```python
from build123d import *

# Parameters (mm, degrees)
SKETCH1_R           = 4
SKETCH1_R_2         = 1.5
BOSS_EXTRUDE1_DEPTH = 5


with BuildPart() as part:
    # Sketch1 → Boss-Extrude1 (new body)
    with BuildSketch(Plane(origin=(0, 0, 0), x_dir=(0, 0, -1), z_dir=(1, 0, 0))):
        Polygon((70.251703358, 12.402398233), (70.251703358, 25.602398233), (65.251703358, 25.602398233), (65.251703358, 33.602398233), (-99.748296642, 33.602398233), (-99.748296642, 25.602398233), (-104.748296642, 25.602398233), (-104.748296642, 12.402398233), (-99.748296642, 12.402398233), (-99.748296642, 4.702398233), (-88.748296642, 4.702398233), (-88.748296642, 6.002398233), (-86.248296642, 6.002398233), (-86.248296642, 4.702398233), (-79.39106139, 4.702398233), (-79.39106139, 1.702398233), (-86.248296642, 1.702398233), (-86.248296642, 0.402398233), (-88.748296642, 0.402398233), (-88.748296642, 1.702398233), (-99.748296642, 1.702398233), (-99.748296642, -5.997601767), (-104.748296642, -5.997601767), (-104.748296642, -19.197601767), (-99.748296642, -19.197601767), (-99.748296642, -27.197601767), (65.251703358, -27.197601767), (65.251703358, -19.197601767), (70.251703358, -19.197601767), (70.251703358, -5.997601767), (65.251703358, -5.997601767), (65.251703358, 1.702398233), (54.251703358, 1.702398233), (54.251703358, 0.402398233), (51.751703358, 0.402398233), (51.751703358, 1.702398233), (44.894468105, 1.702398233), (44.894468105, 4.702398233), (51.751703358, 4.702398233), (51.751703358, 6.002398233), (54.251703358, 6.002398233), (54.251703358, 4.702398233), (65.251703358, 4.702398233), (65.251703358, 12.402398233), align=None)
        with Locations((-17.248296642, 3.202398233)):
            Circle(SKETCH1_R, mode=Mode.SUBTRACT)
        with Locations((-26.248296642, 3.202398233)):
            Circle(SKETCH1_R_2, mode=Mode.SUBTRACT)
        with Locations((-8.248296642, 3.202398233)):
            Circle(SKETCH1_R_2, mode=Mode.SUBTRACT)
    extrude(amount=BOSS_EXTRUDE1_DEPTH)


solid = part.part
```
Geometry check sheet. Reference: the model listing, model coordinates, mm. A direction names the side the tool comes from. Give positions to 0.01 mm unless a question says otherwise; leave off trailing zeros. Order: outer loops, then holes, each group sorted by start corner. A loop starts at its lowest first (then second) coordinate and runs counter-clockwise, first axis right, second up.
1. Gauge pin test, flat ends, axial feed: pin 1 Ø5 at (y, z) = (3.2, 17.25) entering from -X; pin 2 Ø0.6 at (x, y) = (3, 5.5) entering from +Z; pin 3 Ø1 at (x, y) = (2, 0) entering from -Z; pin 4 Ø2.5 at (x, y) = (3.5, 3) entering from -Z. Record the tip position at first contact, or that the pin passes through.
2. Release check for a two-part mould opening along Y. For faces 1 (the face through (2, -27.198, 18)), 2 (the face through (2, 1.702, -48)), 3 (the face through (2, 3, 79.391)), 4 (the face through (0, 10, 18)) record: pulls with the +Y half, pulls with the -Y half, needs draft (parallel to the pull), parting line crosses it, or undercut.
3. Thickness scan on L1, parallel to Z at x = 2.4, y = 3.5; L2, parallel to Y at x = 1.8, z = 26; L3, parallel to Z at x = 4.7, y = 0.5. Record the ranges inside material, lowest first.
4. Section check A-A, the plane z = 91. Enter the section's corners in (x, y), and give its area (3 significant figures).
5. Section check B-B, the plane y = 10.5. Enter the section's corners in (x, z), and give its area (3 significant figures).
6. Section check C-C, the plane x = 3.9. Give the number of separate pieces and of enclosed holes in the cut face, and give its area (3 significant figures).
7. Access from +Z, -Z, +X, -X, +Y, -Y to the whole of each face (thin tool, end or side, straight path). Record for faces 5 (the face through (2, 30, -65.252)), 6 (the face through (2, 12.402, 102)), 7 (the face through (2, 4.702, -60)).
Values follow:
1. pin 1: passes through
1. pin 2: stops at z = 99.75
1. pin 3: stops at z = -65.25
1. pin 4: stops at z = -44.89
2. face 1: pulls with the -Y half
2. face 2: undercut
2. face 3: undercut
2. face 4: needs draft
3. L1: z = -44.89 to 6.78, 9.72 to 13.26, 21.24 to 24.78, 27.72 to 79.39
3. L2: y = -27.2 to 1.72, 4.68 to 33.6
3. L3: z = -65.25 to -54.25, -51.75 to 14.3, 20.2 to 86.25, 88.75 to 99.75
4. outline: (0, -27.2) - (5, -27.2) - (5, 1.7) - (0, 1.7) - close; (0, 4.7) - (5, 4.7) - (5, 33.6) - (0, 33.6) - close
4. area: 289 mm2
5. outline: (0, -65.25) - (5, -65.25) - (5, 99.75) - (0, 99.75) - close
5. area: 825 mm2
6. separate pieces: 1
6. enclosed holes: 3
6. area: 10,100 mm2
7. face 5: -Z, +X, -X, +Y
7. face 6: +Z, +X, -X
7. face 7: -Z, +X, -X
